Here's how the part is built. I have some questions about the finished solid (model axes, mm). Face numbers are marked on the shaded views. A direction names the side the tool comes from. Coordinates: 2 decimals unless noted, no trailing zeros. Loops run counter-clockwise (first coordinate to the right, second up) from the corner with the lowest first, then second, coordinate; pieces in that order, holes last.
from build123d import *

# Parameters (mm, degrees)
EXTRUDE_1_DEPTH     = 10
CHAMFER_1_SIZE      = 2
CUT_EXTRUDE_1_DEPTH = 5
SKETCH_5_R          = 32.43595028
SKETCH_5_R_2        = 6
CUT_EXTRUDE_2_DEPTH = 3
CUT_EXTRUDE_3_DEPTH = 4
SKETCH_7_W          = 54.061660739
SKETCH_7_H          = 47.527586942
SKETCH_7_R          = 4
CUT_EXTRUDE_4_DEPTH = 1
CHAMFER_2_SIZE      = 1


with BuildPart() as part:
    # 草图1 → 凸台-拉伸1 (new body)
    with BuildSketch(Plane(origin=(0, 0, 0), x_dir=(1, 0, 0), z_dir=(0, 1, 0))):
        with BuildLine():
            Line((0, 6), (19, 6))
            ThreePointArc((19, 6), (25, 0), (19, -6))
            Line((19, -6), (0, -6))
            ThreePointArc((0, -6), (-6, 0), (0, 6))
        make_face()
    extrude(amount=EXTRUDE_1_DEPTH)

    # 草图2 → 切除-旋转1 (revolve, cut)
    with BuildSketch(Plane.XY, mode=Mode.PRIVATE) as cut_revolve_1_sk:
        Polygon((0, 10), (-2.8, 10), (-2.8, 5), (-1.85, 5), (-1.85, 2), (-2.8, 2), (-2.8, 0), (0, 0), align=None)
    revolve(cut_revolve_1_sk.sketch.rotate(Axis((0, -1.427566958, 0), (0, 1, 0)), 270), axis=Axis((0, -1.427566958, 0), (0, 1, 0)), mode=Mode.SUBTRACT)

    # 草图3 → 切除-旋转2 (revolve, cut)
    with BuildSketch(Plane.XY, mode=Mode.PRIVATE) as cut_revolve_2_sk:
        Polygon((19, 0), (16.675, 0), (16.675, 6), (16.25, 6), (16.25, 10), (19, 10), align=None)
    revolve(cut_revolve_2_sk.sketch.rotate(Axis((19, 0, 0), (0, 1, 0)), 270), axis=Axis((19, 0, 0), (0, 1, 0)), mode=Mode.SUBTRACT)

    # 倒角1
    chamfer_1_edges = [part.edges().sort_by_distance(p)[0] for p in [
        (25, 10, 0),
        (9.5, 10, -6),
        (-6, 10, 0),
        (9.5, 10, 6),
    ]]
    chamfer(chamfer_1_edges, length=CHAMFER_1_SIZE)

    # 草图4 → 切除-拉伸1 (cut)
    with BuildSketch(Plane.XZ):
        Polygon((2.107328483, 3.65), (-2.107328483, 3.65), (-4.214656965, 0), (-2.107328483, -3.65), (2.107328483, -3.65), (4.214656965, 0), align=None)
    extrude(amount=-CUT_EXTRUDE_1_DEPTH, mode=Mode.SUBTRACT)

    # 草图5 → 切除-拉伸2 (cut)
    with BuildSketch(Plane.XZ):
        Circle(SKETCH_5_R)
        with Locations(Location((0, 0, 0), (0, 0, 90))):
            Circle(SKETCH_5_R_2, mode=Mode.SUBTRACT)
    extrude(amount=-CUT_EXTRUDE_2_DEPTH, mode=Mode.SUBTRACT)

    # 草图6 → 切除-拉伸3 (cut)
    with BuildSketch(Plane(origin=(0, 10, 0), x_dir=(1, 0, 0), z_dir=(0, 1, 0))):
        Polygon((20.674315781, 2.9), (17.325684219, 2.9), (15.651368439, 0), (17.325684219, -2.9), (20.674315781, -2.9), (22.348631561, 0), align=None)
    extrude(amount=-CUT_EXTRUDE_3_DEPTH, mode=Mode.SUBTRACT)

    # 草图7 → 切除-拉伸4 (cut)
    with BuildSketch(Plane(origin=(0, 10, 0), x_dir=(1, 0, 0), z_dir=(0, 1, 0))):
        with Locations((6.682015694, 1.141108586)):
            Rectangle(SKETCH_7_W, SKETCH_7_H)
        with Locations(Location((0, 0, 0), (0, 0, 270))):
            Circle(SKETCH_7_R, mode=Mode.SUBTRACT)
        with Locations(Location((19, 0, 0), (0, 0, 270))):
            Circle(SKETCH_7_R, mode=Mode.SUBTRACT)
    extrude(amount=-CUT_EXTRUDE_4_DEPTH, mode=Mode.SUBTRACT)

    # 倒角2
    chamfer_2_edges = [part.edges().sort_by_distance(p)[0] for p in [
        (19, 9, -4),
        (0, 9, -4),
    ]]
    chamfer(chamfer_2_edges, length=CHAMFER_2_SIZE - 0.0001)  # a hair under: the kernel refuses the full size


solid = part.part
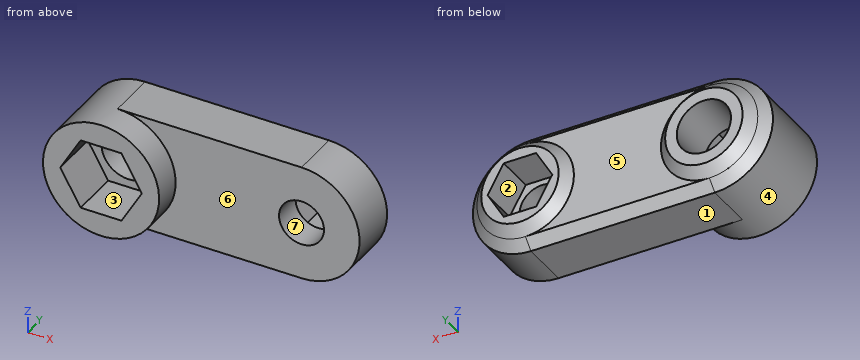
Q1. Suppose I cut it at A-A on y = 9.5. Write out the boundary of the cut face in (x, z).
Q2. Suppose I cut it at B-B on y = 2.25. Write out the boundary of the cut face in (x, z), and give its area (3 significant figures).
Q3. Will these pins go through, and if not, where does the flat tip stop? P1, Ø4, axis at x = 14.5, z = -2, coming from the +Y side; P2, Ø1.5, axis at x = 7, z = -2, coming from the +Y side; P3, Ø6, axis at x = 19, z = 0, coming from the -Y side.
Q4. Suppose I cut it at D-D on z = 2. State how many separate pieces and enclosed holes the cut face has, and give its area (3 significant figures).
Q5. For the marked faces 1, 2 and 3, which set-ups out of +Z, -Z, +X, -X, +Y, -Y let a thin tool reach every point of the face, with its end or its side?
Q6. We'd pull the mould along X, two halves only. Please class the marked faces 4, 5, 6 and 7: pulls with the +X half, pulls with the -X half, needs draft (parallel to the pull), parting line crosses it, or undercut.
Q7. Suppose I cut it at C-C on x = 12.5. Write out the boundary of the cut face in (y, z).
Q8. Please list where these lines run through material, in increasing order: probe 1 along Z at (x, y) = (19, 4.45) (3 decimals); probe 2 along Y at (x, z) = (1, 3.5); probe 3 along Y at (x, z) = (13.5, 2).
Check values:
1. outline: circle Ø9 at (0, 0); circle Ø9 at (19, 0); hole circle Ø5.6 at (0, 0); hole (15.65, 0) - (17.33, -2.9) - (20.67, -2.9) - (22.35, 0) - (20.67, 2.9) - (17.33, 2.9) - close
2. outline: circle Ø12 at (0, 0); hole (-4.21, 0) - (-2.11, -3.65) - (2.11, -3.65) - (4.21, 0) - (2.11, 3.65) - (-2.11, 3.65) - close
2. area: 66.9 mm2
3. P1: stops at y = 10
3. P2: stops at y = 9
3. P3: stops at y = 3
4. separate pieces: 3
4. enclosed holes: 0
4. area: 156 mm2
5. face 1: -Z, +X, -X, +Y, -Y
5. face 2: +Y
5. face 3: -Y
6. face 4: parting line crosses it
6. face 5: undercut
6. face 6: needs draft
6. face 7: undercut
7. outline: (3, -6) - (8, -6) - (9, -5) - (9, 5) - (8, 6) - (3, 6) - close
8. probe 1: z = -6 to -2.325, 2.325 to 6
8. probe 2: y = 5 to 10
8. probe 3: y = 3 to 9
